Autodesk Inventor part; units mm, degrees
ref_plane "YZ Plane" through (0, 0, 0) normal (1, 0, 0) x (0, 1, 0)
ref_plane "XZ Plane" through (0, 0, 0) normal (0, 1, 0) x (-1, 0, 0)
ref_plane "XY Plane" through (0, 0, 0) normal (0, 0, 1) x (1, 0, 0)
sketch "Sketch1" plane through (0, 0, 0) normal (0, 0, 1) x (1, 0, 0)
  line L0 (-30, 19.8) -> (30, 19.8)
  line L1 (30, 19.8) -> (30, 0)
  line L2 (30, 0) -> (-30, 0)
  line L3 (-30, 0) -> (-30, 19.8)
  line L4 (-30, 0) -> (30, 0)
  line L5 (30, 0) -> (30, -15)
  line L6 (30, -15) -> (-30, -15)
  line L7 (-30, -15) -> (-30, 0)
  line L8 (-30, -15) -> (30, -15)
  line L9 (30, -15) -> (30, -20)
  line L10 (30, -20) -> (-30, -20)
  line L11 (-30, -20) -> (-30, -15)
  line L12 (-30, -17.5) -> (30, -17.5)
  line L13 (-40, -15) -> (40, -15)
  line L14 (40, -15) -> (40, -20)
  line L15 (40, -20) -> (-40, -20)
  line L16 (-40, -20) -> (-40, -15)
  line L17 (-40, -15) -> (40, -20) construction
  line L18 (40, -15) -> (-40, -20) construction
  line L19 (0, 0) -> (0, -20)
  point P0 (0, -17.5)
  point P1 (-40, -17.5)
  point P2 (-30, -15)
  dimension "d0" = 60
  dimension "d1" = 19.8
  dimension "d2" = 15
  dimension "d5" = 5
  dimension "d6" = 80
extrude "Extrusion1" add sketch "Sketch1" along normal blind 5 contours L0 L1 L2 L3 | L2 L19 L6 L7 | L5 L6 L19 L2
extrude "Extrusion2" add sketch "Sketch1" along normal blind 30 contours L6 L19 L12 L11 | L11 L15 L16 L13 | L9 L12 L19 L6 | L13 L14 L15 L9 | L12 L19 L10 L11 | L9 L10 L19 L12
sketch "Sketch2" plane through (0, 0, 5) normal (0, 0, 1) x (1, 0, 0)
  line L0 (-30, -15) -> (30, -15)
  line L1 (-29.9232, 0) -> (30, 0)
  line L2 (30, 0) -> (30, -15)
  line L3 (30, -15) -> (-29.9232, -15)
  line L4 (-29.9232, -15) -> (-29.9232, 0)
  line L5 (-30, 19.8) -> (-30, -15)
  line L6 (-30, 4.9) -> (30.0951, 4.9)
  line L7 (-30, 14.9) -> (30, 14.9)
  line L8 (30, -15) -> (30, 19.8)
  line L9 (30, 19.8) -> (-30, 19.8)
  circle A0 centre (-24.89, 4.9) radius 2.5
  circle A1 centre (24.89, 4.9) radius 2.5
  line L10 (-24.89, 4.9) -> (24.89, 4.9)
  line L11 (0, 0) -> (0, 4.9)
  line L12 (-30, 14.9) -> (-30, 4.9)
  line L13 (-30, 9.9) -> (30, 9.9)
  circle A2 centre (-24.89, 14.9) radius 2.5
  circle A3 centre (24.89, 14.9) radius 2.5
  dimension "d9" = 15
  dimension "d10" = 4.9
  dimension "d11" = 4.9
  dimension "d12" = 5
  dimension "d13" = 5
  dimension "d14" = 49.78
  dimension "d15" = 24.89
extrude "Extrusion3" cut sketch "Sketch2" against normal blind 30 contours A0 L6 | L6 A0 | A2 L7 | L7 A2 | A1 L6 | L6 A1 | A3 L7 | L7 A3
properties part number "fp v2 servo Mounting"
Source: CAD feature listing. Evaluate the final solid. Frame: model axes, mm. A direction names the side the tool comes from. Give positions to 0.01 mm unless a question says otherwise; leave off trailing zeros. Write each loop counter-clockwise with the first axis right and the second up, starting at its lowest first coordinate (ties: lowest second). Pieces come first, ordered by that corner, then holes. Notation, with made-up numbers: (58, -31.5) -> (84, -31.5) arc R21 ccw to (84, -26.5) -> close; hole circle Ø3 at (-32, 40.5). An arc over 180 degrees is marked (long way). Write item = value, one per line.
Q1. First-contact query: pin 1 (8 mm diameter, centred on x = -4.5, y = -10.5, fed in from +Z); pin 2 (3 mm diameter, centred on x = -17, y = 14, fed in from -Z); pin 3 (1.5 mm diameter, centred on x = 16, z = 16, fed in from +Y); pin 4 (4 mm diameter, centred on y = 9, z = 3, fed in from -X). Flat tips, straight axial feed; report the tip coordinate or a pass-through.
Here are the results:
pin_1 = 5
pin_2 = 0
pin_3 = -15
pin_4 = -30
Q2. Cut plane B-B on x = 24.89. Return loops of the section in (y, z), then the cut area to 3 significant figures.
Here are the results:
outline = (-20, 0) -> (2.4, 0) -> (2.4, 5) -> (-15, 5) -> (-15, 30) -> (-20, 30) -> close; (7.4, 0) -> (12.4, 0) -> (12.4, 5) -> (7.4, 5) -> close; (17.4, 0) -> (19.8, 0) -> (19.8, 5) -> (17.4, 5) -> close
area = 274 mm²
Q3. Line query: line 1 (X direction, y = 14.9, z = 1.35); line 2 (Y direction, x = -24.89, z = 3.6); line 3 (Z direction, x = -1.5, y = -14.5). Output: solid intervals per line, ascending. Write a range as from..to.
Here are the results:
line_1 = -30..-27.39, -22.39..22.39, 27.39..30
line_2 = -20..2.4, 7.4..12.4, 17.4..19.8
line_3 = 0..5
Q4. Cut plane D-D on z = 23. Return loops of the section in (x, y).
Here are the results:
outline = (-40, -20) -> (40, -20) -> (40, -15) -> (-40, -15) -> close
Q5. Cut plane A-A on y = 14.9. Return loops of the section in (x, z), then the cut area to 3 significant figures.
Here are the results:
outline = (-30, 0) -> (-27.39, 0) -> (-27.39, 5) -> (-30, 5) -> close; (-22.39, 0) -> (22.39, 0) -> (22.39, 5) -> (-22.39, 5) -> close; (27.39, 0) -> (30, 0) -> (30, 5) -> (27.39, 5) -> close
area = 250 mm²
Q6. Mould query, pull axis Y, two halves, no side actions, for faces 6 (the face through (-1, -17, 30)), 7 (the face through (-26.874, 13.379, 2.535)), 8 (the face through (1, -15, 18)), 9 (the face through (1, -20, 15)). Classes: +Y half, -Y half, draft (parallel to the pull), parting line (faces both ways), or undercut.
Here are the results:
face_6 = draft
face_7 = undercut
face_8 = +Y half
face_9 = -Y half
Q7. Cut plane C-C on x = -14. Return loops of the section in (y, z).
Here are the results:
outline = (-20, 0) -> (19.8, 0) -> (19.8, 5) -> (-15, 5) -> (-15, 30) -> (-20, 30) -> close
Q8. Reachability of faces 1 (the face through (0, 3, 5)), 2 (the face through (30, 3, 2)), 3 (the face through (0, 19.8, 2)), 4 (the face through (-30, 2, 2)), 5 (the face through (-26.874, 3.379, 2.535)) from +Z, -Z, +X, -X, +Y, -Y: full face, straight path, thin tool, end or side. Return the list, or none.
Here are the results:
face_1 = +Z, +X, -X, +Y
face_2 = +Z, -Z, +X, +Y
face_3 = +Z, -Z, +X, -X, +Y
face_4 = +Z, -Z, -X, +Y
face_5 = +Z, -Z
